For this review, take the finished solid that the model builds, in its own axes (mm). Coordinates: 2 decimals unless noted, no trailing zeros. Order: outer loops, then holes, each group sorted by start corner. A loop starts at its lowest first (then second) coordinate and runs counter-clockwise, first axis right, second up. Notation, with made-up numbers: (45, 41) -> (97, 41) arc R17 cw to (97, 59) -> close; hole circle Ø10 at (3, 22.25). An arc over 180 degrees is marked (long way). Answer as a JSON object with one key per item and string values. Group by question number.
1) Add section A-A, the plane z = -1.5. Write out the cut boundary in (x, y).
2) Add section B-B, the plane y = -0.6. Write out the cut boundary in (x, z), then the cut area to 3 significant figures.
3) For pin 1 (1 mm diameter, centred on y = -2, z = -14, fed in from -X); pin 2 (1.4 mm diameter, centred on x = -2.5, y = -2, fed in from -Z); pin 3 (1.4 mm diameter, centred on y = -2, z = 8.5, fed in from -X), all flat-tipped, find the tip position at first contact; note any pin that passes through.
4) Wall thickness on L1, parallel to X at y = -1.75, z = 6; L2, parallel to Y at x = -7.5, z = -5; L3, parallel to X at y = -1.4, z = 19: over which ranges is each line inside the solid? List them lowest first.
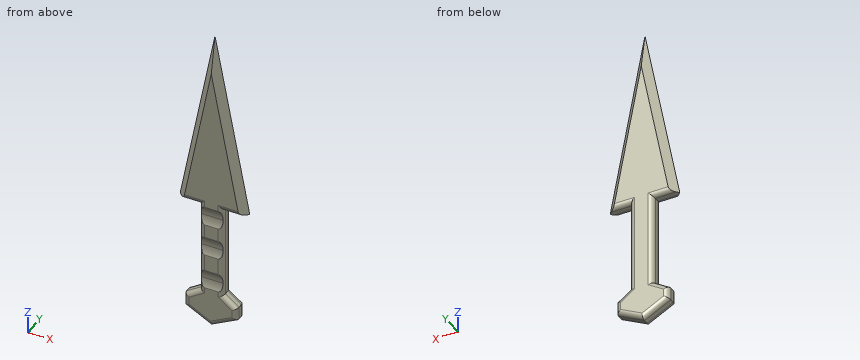
from build123d import *

# Parameters (mm, degrees)
F1_DEPTH = 3.81
F2_SIZE  = 1.90499
F3_R     = 1.27
F5_DEPTH = 25.4


# Not quite as in the source:
# - a fillet or chamfer is up to 0.001 mm smaller than in the source, because OpenCascade refuses the exact size
# - a feature names something its author has since deleted; it is built from what else it names


with BuildPart() as f1:
    # F0 (on Front) → F1 (new body)
    with BuildSketch(Plane.XZ):
        Polygon((-12.1744828463, 16.8822405368), (-12.1744828463, -8.5177594632), (-16.408668831, -11.2550966442), (-16.408668831, -14.7449430078), (-9.2011271045, -18.4709690511), (-2.1051054355, -14.7449430078), (-2.1051054355, -11.2550966442), (-5.8244828463, -8.5177594632), (-5.8244828463, 16.8822405368), (0.5255171537, 16.8822405368), (-8.9994828463, 66.7812823613), (-18.5244828463, 16.8822405368), align=None)
    extrude(amount=F1_DEPTH)

    # F2 (size 1.905 in the source; OpenCascade refuses exactly that, so slightly less here)
    f2_edges = [f1.edges().sort_by_distance(p)[0] for p in [
        (-13.761983, -3.81, 41.831761),
        (-4.236983, -3.81, 41.831761),
        (-13.761983, 0, 41.831761),
        (-4.236983, 0, 41.831761),
    ]]
    chamfer(f2_edges, length=F2_SIZE)

    # F3
    f3_edges = [f1.edges().sort_by_distance(p)[0] for p in [
        (-12.174483, -3.81, 4.182241),
        (-5.824483, -3.81, 4.182241),
        (-12.174483, 0, 4.182241),
        (-5.824483, 0, 4.182241),
        (-14.37979, -3.81, 16.882241),
        (-3.619176, 0, 16.882241),
        (-3.619176, -3.81, 16.882241),
        (-14.37979, 0, 16.882241),
        (-14.291576, -3.81, -9.886428),
        (-16.408669, -3.81, -13.00002),
        (-12.804898, -3.81, -16.607956),
        (-5.653116, -3.81, -16.607956),
        (-2.105105, -3.81, -13.00002),
        (-3.964794, -3.81, -9.886428),
        (-14.291576, 0, -9.886428),
        (-3.964794, 0, -9.886428),
        (-2.105105, 0, -13.00002),
        (-5.653116, 0, -16.607956),
        (-12.804898, 0, -16.607956),
        (-16.408669, 0, -13.00002),
    ]]
    fillet(f3_edges, radius=F3_R)

    # F4 (on Right) → F5 (cut)
    with BuildSketch(Plane.YZ):
        with BuildLine():
            ThreePointArc((-5.1016697734, 9.2693595216), (-3.730698506, 11.3268088009), (-3.2493867144, 13.7518858537))
            ThreePointArc((-3.2493867144, 13.7518858537), (-12.0244637672, 19.6205740621), (-14.0971036554, 9.2693595216))
            ThreePointArc((-14.0971036554, 9.2693595216), (-9.5993867144, 11.1368331894), (-5.1016697734, 9.2693595216))
        make_face()
        with BuildLine():
            ThreePointArc((-5.1016697734, 9.2693595216), (-9.5993867144, 11.1368331894), (-14.0971036554, 9.2693595216))
            ThreePointArc((-14.0971036554, 9.2693595216), (-9.5993867144, 7.4018858537), (-5.1016697734, 9.2693595216))
        make_face()
        with BuildLine():
            ThreePointArc((-5.1016697734, 9.2693595216), (-9.5993867144, 7.4018858537), (-14.0971036554, 9.2693595216))
            ThreePointArc((-14.0971036554, 9.2693595216), (-15.9420131796, 4.4809091421), (-13.6448170782, -0.107754962))
            ThreePointArc((-13.6448170782, -0.107754962), (-9.6056271037, 1.3330596991), (-5.571670106, -0.1223417843))
            ThreePointArc((-5.571670106, -0.1223417843), (-3.8592429678, 2.0714603295), (-3.2493867144, 4.7868331894))
            ThreePointArc((-3.2493867144, 4.7868331894), (-3.730698506, 7.2119102423), (-5.1016697734, 9.2693595216))
        make_face()
        with BuildLine():
            ThreePointArc((-5.571670106, -0.1223417843), (-9.6108600804, -1.5631564454), (-13.6448170782, -0.107754962))
            ThreePointArc((-13.6448170782, -0.107754962), (-12.3324733297, -10.7570736823), (-3.2671004698, -5.0169299357))
            ThreePointArc((-3.2671004698, -5.0169299357), (-3.8720598777, -2.311932968), (-5.571670106, -0.1223417843))
        make_face()
        with BuildLine():
            ThreePointArc((-5.571670106, -0.1223417843), (-9.6056271037, 1.3330596991), (-13.6448170782, -0.107754962))
            ThreePointArc((-13.6448170782, -0.107754962), (-9.6108600804, -1.5631564454), (-5.571670106, -0.1223417843))
        make_face()
    extrude(amount=-F5_DEPTH, mode=Mode.SUBTRACT)


solid = f1.part
Output values:
{
 "1": {"outline": "(-12.17, -2.54) arc R1.27 ccw to (-10.9, -3.81) -> (-7.09, -3.81) arc R1.27 ccw to (-5.82, -2.54) -> (-5.82, -1.27) arc R1.27 ccw to (-7.09, 0) -> (-10.9, 0) arc R1.27 ccw to (-12.17, -1.27) -> close"},
 "2": {"outline": "(-17.16, 17.07) -> (-11.98, 17.07) -> (-11.98, -8.62) -> (-16.22, -11.36) -> (-16.22, -14.63) -> (-9.2, -18.26) -> (-2.3, -14.63) -> (-2.3, -11.35) -> (-6.02, -8.61) -> (-6.02, 17.07) -> (-0.84, 17.07) -> (-9, 59.82) -> close", "area": "600 mm²"},
 "3": {"pin 1": "stops at x = -16.41", "pin 2": "stops at z = -15.32", "pin 3": "stops at x = -12.17"},
 "4": {"L1": "x = -12.17 to -5.82", "L2": "y = -3.27 to 0", "L3": "x = -17.61 to -0.39"}
}
